The listing builds one solid part. Answer for the finished solid, in the listing's coordinates (mm). Coordinates: 2 decimals unless noted, no trailing zeros. Write each loop counter-clockwise with the first axis right and the second up, starting at its lowest first coordinate (ties: lowest second). Pieces come first, ordered by that corner, then holes.
from build123d import *

# Parameters (mm, degrees)
SKETCH1_W           = 140
SKETCH1_H           = 80
BOSS_EXTRUDE1_DEPTH = 4
SKETCH2_R           = 6.675
SKETCH2_R_2         = 1.7
SKETCH2_R_3         = 15
CUT_EXTRUDE1_DEPTH  = 4
FILLET1_R           = 2


with BuildPart() as part:
    # Sketch1 → Boss-Extrude1 (new body)
    with BuildSketch(Plane.XY):
        with Locations((68.890553518, -1.461144776)):
            Rectangle(SKETCH1_W, SKETCH1_H)
    extrude(amount=BOSS_EXTRUDE1_DEPTH)

    # Sketch2 → Cut-Extrude1 (cut)
    with BuildSketch(Plane(origin=(0, 0, 0), x_dir=(-1, 0, 0), z_dir=(0, 0, -1))):
        with Locations((-33.890553518, -1.461144776)):
            Circle(SKETCH2_R)
        with Locations((-33.890553518, 14.758855224)):
            Circle(SKETCH2_R_2)
        with Locations((-33.890553518, -17.681144776)):
            Circle(SKETCH2_R_2)
        with Locations((-3.890553518, -36.461144776)):
            Circle(SKETCH2_R_2)
        with Locations((-133.890553518, -36.461144776)):
            Circle(SKETCH2_R_2)
        with Locations((-133.890553518, 33.538855224)):
            Circle(SKETCH2_R_2)
        with Locations((-3.890553518, 33.538855224)):
            Circle(SKETCH2_R_2)
        with Locations((-102.890553518, -1.461144776)):
            Circle(SKETCH2_R_3)
    extrude(amount=-CUT_EXTRUDE1_DEPTH, mode=Mode.SUBTRACT)

    # Fillet1
    fillet1_edges = [part.edges().sort_by_distance(p)[0] for p in [
        (-1.109446482, 38.538855224, 2),
        (138.890553518, 38.538855224, 2),
        (138.890553518, -41.461144776, 2),
        (-1.109446482, -41.461144776, 2),
    ]]
    fillet(fillet1_edges, radius=FILLET1_R)


solid = part.part
1. Section B-B on x = 113.5 is taken. Give the vertices of the cut face in (y, z).
Results found:
outline: (-41.46, 0) - (-12.06, 0) - (-12.06, 4) - (-41.46, 4) - close; (9.14, 0) - (38.54, 0) - (38.54, 4) - (9.14, 4) - close
2. For a pull along X with two mould halves and no side action, classify faces 1 (the cylindrical face through (117.876, -0.802, 1.972)), 2 (the flat face through (-1.109, -2, 2)), 3 (the flat face through (68, -1, 0)) as pulls with the +X half, pulls with the -X half, needs draft (parallel to the pull), parting line crosses it, or undercut.
Results found:
face 1: undercut
face 2: pulls with the -X half
face 3: needs draft
3. Section A-A on y = 9 is taken. Give the vertices of the cut face in (x, z), then the cut area to 3 significant figures.
Results found:
outline: (-1.11, 0) - (92.14, 0) - (92.14, 4) - (-1.11, 4) - close; (113.64, 0) - (138.89, 0) - (138.89, 4) - (113.64, 4) - close
area: 474 mm2
4. Find the intervals of material crossed by L1, parallel to X at y = 34, z = 1.2; L2, parallel to Y at x = 33, z = 3.45; L3, parallel to X at y = -7.5, z = 3, in increasing order.
Results found:
L1: x = -1.11 to 2.25, 5.53 to 132.25, 135.53 to 138.89
L2: y = -41.46 to -19.13, -16.23 to -8.08, 5.15 to 13.31, 16.21 to 38.54
L3: x = -1.11 to 31.05, 36.73 to 89.16, 116.62 to 138.89
5. Section C-C on z = 1.8 is taken. State how many separate pieces and enclosed holes the cut face has, then the cut area to 3 significant figures.
Results found:
separate pieces: 1
enclosed holes: 8
area: 10,300 mm2
6. A flat-ended cylindrical pin translates along its axis: P1, Ø2, axis at x = 33.89, y = 14.76, coming from the +Z side (1 decimal). Find the tip coordinate at first contact, or state that the pin passes through.
Results found:
P1: passes through
